```python
from build123d import *

# Parameters (mm, degrees)
SKETCH1_R           = 2.5
BOSS_EXTRUDE1_DEPTH = 5
SKETCH2_W           = 5
SKETCH2_H           = 20
BOSS_EXTRUDE2_DEPTH = 40
BOSS_EXTRUDE3_DEPTH = 5
BOSS_EXTRUDE4_DEPTH = 5


with BuildPart() as part:
    # Sketch1 → Boss-Extrude1 (new body)
    with BuildSketch(Plane.XY):
        with BuildLine():
            Line((-15, -10), (-15, 10))
            Line((-15, 10), (15, 10))
            ThreePointArc((15, 10), (25, 0), (15, -10))
            Line((15, -10), (-15, -10))
        make_face()
        with Locations((15, 0)):
            Circle(SKETCH1_R, mode=Mode.SUBTRACT)
    extrude(amount=BOSS_EXTRUDE1_DEPTH)

    # Sketch2 → Boss-Extrude2 (add)
    with BuildSketch(Plane(origin=(0, 0, 0), x_dir=(-1, 0, 0), z_dir=(0, 0, -1))):
        with Locations((12.5, 0)):
            Rectangle(SKETCH2_W, SKETCH2_H)
    extrude(amount=BOSS_EXTRUDE2_DEPTH)

    # Sketch4 → Boss-Extrude3 (add)
    with BuildSketch(Plane.XZ.offset(10)):
        Polygon((-10, -20), (10, 0), (-10, 0), align=None)
    extrude(amount=-BOSS_EXTRUDE3_DEPTH)

    # Sketch5 → Boss-Extrude4 (add)
    with BuildSketch(Plane(origin=(0, 10, 0), x_dir=(1, 0, 0), z_dir=(0, 1, 0))):
        Polygon((10, 0), (-10, 20), (-10, 0), align=None)
    extrude(amount=-BOSS_EXTRUDE4_DEPTH)


solid = part.part
```
Verification items for the finished model (mm, model axes). A direction names the side the tool comes from. Coordinates: 2 decimals unless noted, no trailing zeros. Order: outer loops, then holes, each group sorted by start corner. A loop starts at its lowest first (then second) coordinate and runs counter-clockwise, first axis right, second up. Notation, with made-up numbers: (64.5, 48.5) -> (104.5, 48.5) arc R19 cw to (104.5, 65.5) -> close; hole circle Ø5 at (45.5, 62.25). An arc over 180 degrees is marked (long way). Put each result on its own line as item: value. Start each with the question number.
1) Cross-section at C-C (z = -10). Enter the section's corners in (x, y).
2) Cross-section at D-D (z = 1.5). Enter the section's corners in (x, y).
3) Go/stop test with flat-tipped pins: pin 1 (4 mm diameter, centred on x = 7, y = -4.5, fed in from -Z); pin 2 (6 mm diameter, centred on y = 0, z = -13.5, fed in from +X); pin 3 (2 mm diameter, centred on x = -8.5, y = 6, fed in from -Z). Record where each tip stops, or that it passes through.
4) Cross-section at A-A (y = 0). Enter the section's corners in (x, z).
5) Cross-section at B-B (x = -2.5). Enter the section's corners in (y, z), plus the area to 3 significant figures.
6) Material ranges on L1, parallel to Y at x = 15, z = 3.4; L2, parallel to Z at x = 1, y = 3; L3, parallel to X at y = 1.5, z = -36, recorded low to high.
7) Tool access check on faces 1 (the flat face through (-7, 10, -13)), 2 (the flat face through (-2, -5, -8)). Record the directions out of +Z, -Z, +X, -X, +Y, -Y that give a thin tool (end or side, any length) a straight path to the whole face; none if there is none.
Geometry check:
1. outline: (-15, -10) -> (0, -10) -> (0, -5) -> (-10, -5) -> (-10, 5) -> (0, 5) -> (0, 10) -> (-15, 10) -> close
2. outline: (-15, -10) -> (15, -10) arc R10 ccw to (15, 10) -> (-15, 10) -> close; hole circle Ø5 at (15, 0)
3. pin 1: stops at z = -4.94
3. pin 2: stops at x = -10
3. pin 3: stops at z = -19.5
4. outline: (-15, -40) -> (-10, -40) -> (-10, 0) -> (12.5, 0) -> (12.5, 5) -> (-15, 5) -> close; (17.5, 0) -> (25, 0) -> (25, 5) -> (17.5, 5) -> close
5. outline: (-10, -12.5) -> (-5, -12.5) -> (-5, 0) -> (5, 0) -> (5, -12.5) -> (10, -12.5) -> (10, 5) -> (-10, 5) -> close
5. area: 225 mm^2
6. L1: y = -10 to -2.5, 2.5 to 10
6. L2: z = 0 to 5
6. L3: x = -15 to -10
7. face 1: +Z, -Z, +X, -X, +Y
7. face 2: -Z, +X
